```python
from build123d import *

# Parameters (mm, degrees)
CROQUIS1_W                   = 112
CROQUIS1_H                   = 112
CROQUIS1_W_2                 = 96
CROQUIS1_H_2                 = 96
SALIENTE_EXTRUIR2_DEPTH      = 28
CROQUIS2_R                   = 5.155
CORTAR_EXTRUIR1_DEPTH        = 8
CROQUIS3_R                   = 11.115
CORTAR_EXTRUIR2_DEPTH        = 5
CROQUIS4_R                   = 6.5
CORTAR_EXTRUIR3_DEPTH        = 5
SALIENTE_EXTRUIR3_DEPTH      = 28
SALIENTE_EXTRUIR3_DEPTH_BACK = 28
CROQUIS5_W                   = 12
CROQUIS5_H                   = 12


with BuildPart() as part:
    # Croquis1 → Saliente-Extruir2 (new body)
    with BuildSketch(Plane.XY):
        with Locations((32.5, 32.5)):
            Rectangle(CROQUIS1_W, CROQUIS1_H)
        with Locations((32.5, 32.5)):
            Rectangle(CROQUIS1_W_2, CROQUIS1_H_2, mode=Mode.SUBTRACT)
    extrude(amount=-SALIENTE_EXTRUIR2_DEPTH)

    # Croquis2 → Cortar-Extruir1 (cut)
    with BuildSketch(Plane.XZ.offset(23.5)):
        with Locations(Location((32.5, -14, 0), (0, 0, 270))):
            Circle(CROQUIS2_R)
    extrude(amount=-CORTAR_EXTRUIR1_DEPTH, mode=Mode.SUBTRACT)

    # Croquis3 → Cortar-Extruir2 (cut)
    with BuildSketch(Plane.XZ.offset(23.5)):
        with Locations(Location((32.5, -14, 0), (0, 0, 270))):
            Circle(CROQUIS3_R)
    extrude(amount=-CORTAR_EXTRUIR2_DEPTH, mode=Mode.SUBTRACT)

    # Croquis4 → Cortar-Extruir3 (cut)
    with BuildSketch(Plane.XZ.offset(-80.5)):
        with Locations(Location((32.5, -14, 0), (0, 0, 270))):
            Circle(CROQUIS4_R)
    extrude(amount=-CORTAR_EXTRUIR3_DEPTH, mode=Mode.SUBTRACT)

    # Croquis5 → Saliente-Extruir3 (add, two sides: drawn at the far end of the back side and taken through both)
    with BuildSketch(Plane.XY.offset(-SALIENTE_EXTRUIR3_DEPTH_BACK)):
        with Locations((-17.5, 82.5)):
            Rectangle(CROQUIS5_W, CROQUIS5_H)
        with Locations((-17.5, -17.5)):
            Rectangle(CROQUIS5_W, CROQUIS5_H)
        with Locations((82.5, -17.5)):
            Rectangle(CROQUIS5_W, CROQUIS5_H)
        with Locations((82.5, 82.5)):
            Rectangle(CROQUIS5_W, CROQUIS5_H)
    extrude(amount=SALIENTE_EXTRUIR3_DEPTH + SALIENTE_EXTRUIR3_DEPTH_BACK)


solid = part.part
```
Model file for the job. Use its own axes, mm. A direction names the side the tool comes from. Give positions to 0.01 mm unless a question says otherwise; leave off trailing zeros. Loops run counter-clockwise (first coordinate to the right, second up) from the corner with the lowest first, then second, coordinate; pieces in that order, holes last. Notation, with made-up numbers: (-6.75, -22) -> (13.25, -22) arc R24 ccw to (13.25, -3) -> close; hole circle Ø5 at (-15, -3.75). An arc over 180 degrees is marked (long way). Use CSV: the item, a comma, the result in double quotes. Start each with the question number.
1) Tool access for faces 1 (the flat face through (32, -15.5, -20)), 2 (the flat face through (30, -18.5, -19)), 3 (the flat face through (32, 85, 0)), 4 (the flat face through (19, -23.5, -6)), 5 (the flat face through (-11.5, 81, 6)): list every direction of +Z, -Z, +X, -X, +Y, -Y with a clear straight run to the whole face (end or side of a thin tool).
2) Flat gauge pins, fed straight in: pin 1 Ø4 at (x, y) = (86, 17) entering from +Z; pin 2 Ø4 at (x, z) = (34, -13.5) entering from -Y. Where does each tip first touch, or does it go through?
3) Slice it at A-A on y = -1. Give the cut face in (x, z), plus the area to 3 significant figures.
4) Mould opens along X. For faces 6 (the flat face through (32, -19, 0)), 7 (the flat face through (-18, 33, -28)), 8 (the flat face through (-23.5, 32, -12)) say: released by +X, released by -X, zero draft, split by the parting line, or undercut.
5) Slice it at D-D on z = -14. Give the cut face in (x, y) (3 decimals), plus the area to 3 significant figures.
6) Slice it at C-C on x = 32.5. Give the cut face in (y, z) (3 decimals), plus the area to 3 significant figures.
7) Wall check: line 1 (X direction, y = 82.75, z = -14); line 2 (X direction, y = 66.5, z = -24.5); line 3 (Y direction, x = 83.5, z = 19.5). Give the ranges that are in metal, low to high.
Computed values:
1,face 1,"+Z, -Z"
1,face 2,"-Y"
1,face 3,"+Z, +Y, -Y"
1,face 4,"+Z, -Z, +X, -X, -Y"
1,face 5,"+Z"
2,pin 1,"stops at z = 0"
2,pin 2,"stops at y = 85.5"
3,outline,"(-23.5, -28) -> (-15.5, -28) -> (-15.5, 0) -> (-23.5, 0) -> close; (80.5, -28) -> (88.5, -28) -> (88.5, 0) -> (80.5, 0) -> close"
3,area,"448 mm^2"
4,face 6,"undercut"
4,face 7,"zero draft"
4,face 8,"released by -X"
5,outline,"(-23.5, -23.5) -> (21.385, -23.5) -> (21.385, -18.5) -> (27.345, -18.5) -> (27.345, -15.5) -> (-11.5, -15.5) -> (-11.5, -11.5) -> (-15.5, -11.5) -> (-15.5, 76.5) -> (-11.5, 76.5) -> (-11.5, 80.5) -> (26, 80.5) -> (26, 85.5) -> (39, 85.5) -> (39, 80.5) -> (76.5, 80.5) -> (76.5, 76.5) -> (80.5, 76.5) -> (80.5, -11.5) -> (76.5, -11.5) -> (76.5, -15.5) -> (37.655, -15.5) -> (37.655, -18.5) -> (43.615, -18.5) -> (43.615, -23.5) -> (88.5, -23.5) -> (88.5, 88.5) -> (-23.5, 88.5) -> close"
5,area,"3,180 mm^2"
6,outline,"(-23.5, -28) -> (-15.5, -28) -> (-15.5, -19.155) -> (-18.5, -19.155) -> (-18.5, -25.115) -> (-23.5, -25.115) -> close; (-23.5, -2.885) -> (-18.5, -2.885) -> (-18.5, -8.845) -> (-15.5, -8.845) -> (-15.5, 0) -> (-23.5, 0) -> close; (80.5, -28) -> (88.5, -28) -> (88.5, 0) -> (80.5, 0) -> (80.5, -7.5) -> (85.5, -7.5) -> (85.5, -20.5) -> (80.5, -20.5) -> close"
6,area,"241 mm^2"
7,line 1,"x = -23.5 to 26, 39 to 88.5"
7,line 2,"x = -23.5 to -15.5, 80.5 to 88.5"
7,line 3,"y = -23.5 to -11.5, 76.5 to 88.5"
